```python
from build123d import *

# Parameters (mm, degrees)
F0_W     = 939.8
F0_H     = 63.5
F1_DEPTH = 25.4
F2_W     = 939.8
F2_H     = 19.05
F3_DEPTH = 6.35
F4_R     = 1.5875
F5_DEPTH = 25.401


with BuildPart() as f1:
    # F0 (on Front) → F1 (new body)
    with BuildSketch(Plane.XZ):
        with Locations((469.9, -31.75)):
            Rectangle(F0_W, F0_H)
    extrude(amount=-F1_DEPTH)

    # F2 (on Front) → F3 (cut)
    with BuildSketch(Plane.XZ):
        with Locations((469.9, -47.625)):
            Rectangle(F2_W, F2_H)
    extrude(amount=-F3_DEPTH, mode=Mode.SUBTRACT)

    # F4 (on Front) → F5 (cut, through all)
    with BuildSketch(Plane.XZ):
        with Locations((12.7, -47.625)):
            Circle(F4_R)
        with Locations((114.3, -47.625)):
            Circle(F4_R)
        with Locations((215.9, -47.625)):
            Circle(F4_R)
        with Locations((317.5, -47.625)):
            Circle(F4_R)
        with Locations((419.1, -47.625)):
            Circle(F4_R)
        with Locations((520.7, -47.625)):
            Circle(F4_R)
        with Locations((622.3, -47.625)):
            Circle(F4_R)
        with Locations((723.9, -47.625)):
            Circle(F4_R)
        with Locations((825.5, -47.625)):
            Circle(F4_R)
        with Locations((927.1, -47.625)):
            Circle(F4_R)
    extrude(amount=-F5_DEPTH, mode=Mode.SUBTRACT)


solid = f1.part
```
Work out the finished part from the listing and answer in its coordinate system (mm). A direction names the side the tool comes from. Give positions to 0.01 mm unless a question says otherwise; leave off trailing zeros. Write each loop counter-clockwise with the first axis right and the second up, starting at its lowest first coordinate (ties: lowest second). Pieces come first, ordered by that corner, then holes. Notation, with made-up numbers: (5, 43.5) -> (62, 43.5) arc R4 ccw to (62, 50.5) -> close; hole circle Ø10 at (37.25, 27.25). An arc over 180 degrees is marked (long way). Write each question's results on one line, items separated by ' | '.
1. Find section A-A on x = 175. Determine the outline of the cut face in (y, z), and give its area (3 significant figures).
Data:
outline: (0, -63.5) -> (25.4, -63.5) -> (25.4, 0) -> (0, 0) -> (0, -38.1) -> (6.35, -38.1) -> (6.35, -57.15) -> (0, -57.15) -> close | area: 1,490 mm^2
2. Straight lines are drawn through the part: L1, parallel to Z at x = 304, y = 2; L2, parallel to Z at x = 12.7, y = 17.75; L3, parallel to Y at x = 354, z = -48. For each, find the intervals that lie inside material, in ascending order.
Data:
L1: -63.5 to -57.15, -38.1 to 0 | L2: -63.5 to -49.21, -46.04 to 0 | L3: 6.35 to 25.4
3. A tool of negligible diameter and unlimited length cuts with its end or side. For faces 1 (the flat face through (463, 13, 0)), 2 (the flat face through (463, 6.35, -47)), from which of +Z, -Z, +X, -X, +Y, -Y can it reach the whole face along a straight path? Write none if from no direction.
Data:
face 1: +Z, +X, -X, +Y, -Y | face 2: +X, -X, -Y
4. Each of these flat-tipped pins is pushed along its axis until it touches: pin 1 Ø5 at (x, y) = (205.5, 3.5) entering from +Z; pin 2 Ø4 at (x, z) = (114.3, -47.625) entering from -Y; pin 3 Ø2.5 at (x, z) = (520.7, -47.625) entering from +Y. Where does it stop, or does it pass through?
Data:
pin 1: z = 0 | pin 2: y = 6.35 | pin 3: through
